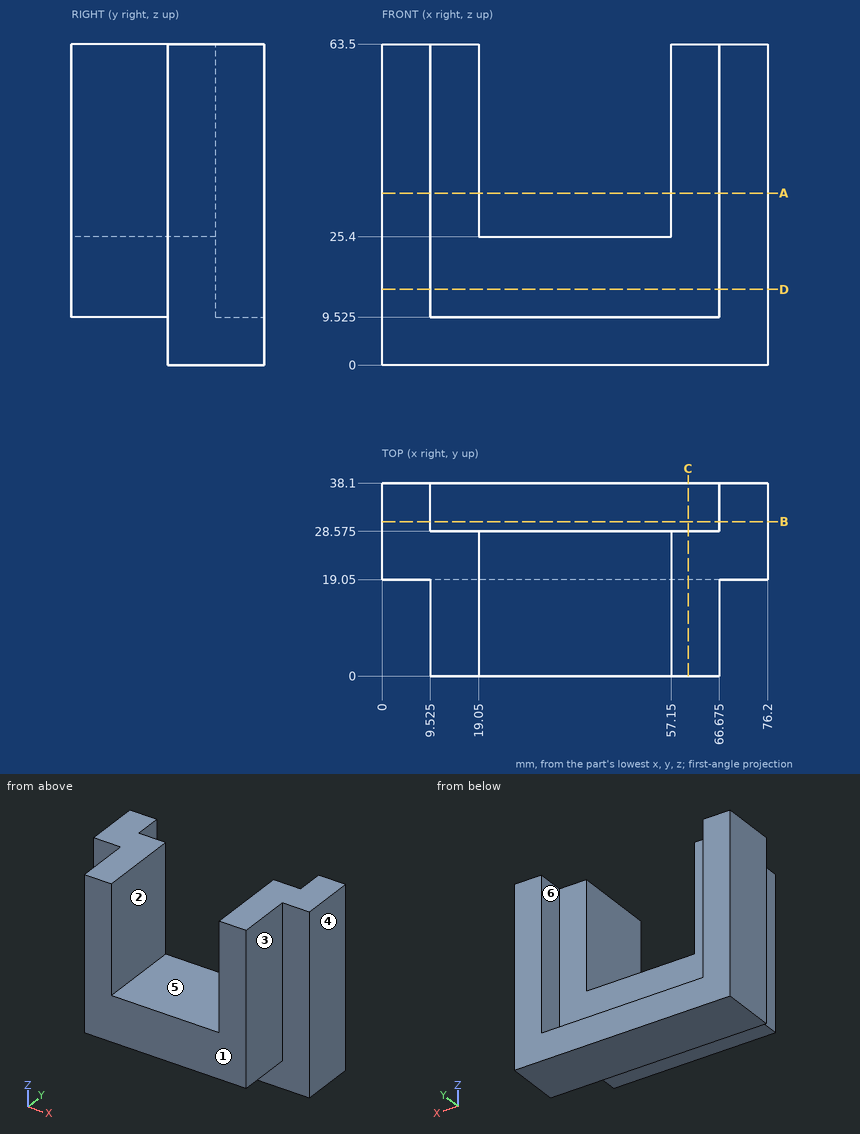
Could you check a few things on this drawing? It's one solid part, dimensions in mm from its lowest x, y, z. A direction names the side the tool comes from. Coordinates: 2 decimals unless noted, no trailing zeros. Loops run counter-clockwise (first coordinate to the right, second up) from the corner with the lowest first, then second, coordinate; pieces in that order, holes last. Notation, with made-up numbers: (24, 51.5) - (39, 51.5) arc R16 cw to (39, 76.5) - close; hole circle Ø2 at (53, 2). An arc over 180 degrees is marked (long way). Answer as a JSON object with one key per item and string values. Group by question number.
Item 1: For pin 1 (5 mm diameter, centred on y = 15.5, z = 45, fed in from -X) (3 decimals); pin 2 (7.5 mm diameter, centred on x = 49, y = 31.5, fed in from +Z); pin 3 (9.5 mm diameter, centred on y = 13, z = 46.5, fed in from +X) (3 decimals), each with a flat end and sliding along its axis, tell me the tip position at first contact or that it passes through.
Item 2: If we section it at C-C (x = 60.5): List the corners of the cut face in (y, z) for me (3 decimals), plus the area to 3 significant figures.
Item 3: If we section it at A-A (z = 34): List the corners of the cut face in (x, y) for me (3 decimals).
Item 4: If we mould it in two halves opening along X, with no side actions, what happens to the marked faces 1, 2 and 3? For each: released by +X, released by -X, zero draft, split by the parting line, or undercut.
Item 5: If we section it at B-B (y = 30.5): List the corners of the cut face in (x, z) for me (3 decimals), plus the area to 3 significant figures.
Item 6: On a 3-axis mill with a long thin cutter (end or side, diameter ignored), from which of +Z, -Z, +X, -X, +Y, -Y can I reach the whole of each face in a straight line? I mean the marked faces 4, 5 and 6. Say none if no direction works.
Item 7: If we section it at D-D (z = 15): List the corners of the cut face in (x, y) for me (3 decimals).
Item 8: If I drill on L1, parallel to X at y = 12, z = 45 (3 decimals); L2, parallel to X at y = 29, z = 29 (3 decimals); L3, parallel to Z at x = 35, y = 23, over which ranges is the centre line in solid material (lowest first)? Write a range as from..to.
Returned:
{
 "1": {"pin 1": "stops at x = 9.525", "pin 2": "stops at z = 25.4", "pin 3": "stops at x = 66.675"},
 "2": {"outline": "(0, 9.525) - (19.05, 9.525) - (19.05, 0) - (38.1, 0) - (38.1, 9.525) - (28.575, 9.525) - (28.575, 63.5) - (0, 63.5) - close", "area": "1,720 mm²"},
 "3": {"outline": "(0, 19.05) - (9.525, 19.05) - (9.525, 0) - (19.05, 0) - (19.05, 28.575) - (9.525, 28.575) - (9.525, 38.1) - (0, 38.1) - close; (57.15, 0) - (66.675, 0) - (66.675, 19.05) - (76.2, 19.05) - (76.2, 38.1) - (66.675, 38.1) - (66.675, 28.575) - (57.15, 28.575) - close"},
 "4": {"face 1": "zero draft", "face 2": "undercut", "face 3": "released by +X"},
 "5": {"outline": "(0, 0) - (76.2, 0) - (76.2, 63.5) - (66.675, 63.5) - (66.675, 9.525) - (9.525, 9.525) - (9.525, 63.5) - (0, 63.5) - close", "area": "1,750 mm²"},
 "6": {"face 4": "+Z, -Z, +X, +Y, -Y", "face 5": "+Z, +Y, -Y", "face 6": "+Z, +Y"},
 "7": {"outline": "(0, 19.05) - (9.525, 19.05) - (9.525, 0) - (66.675, 0) - (66.675, 19.05) - (76.2, 19.05) - (76.2, 38.1) - (66.675, 38.1) - (66.675, 28.575) - (9.525, 28.575) - (9.525, 38.1) - (0, 38.1) - close"},
 "8": {"L1": "x = 9.525..19.05, 57.15..66.675", "L2": "x = 0..9.525, 66.675..76.2", "L3": "z = 0..25.4"}
}
